Model file for the job. Use its own axes, mm. Give positions to 0.01 mm unless a question says otherwise; leave off trailing zeros. Loops run counter-clockwise (first coordinate to the right, second up) from the corner with the lowest first, then second, coordinate; pieces in that order, holes last. Notation, with made-up numbers: M -30,-19 L 10,-19 A11 cw 10,-14 Z; hole C 78,-34 d10. An arc over 180 degrees is marked long. Use CSV: the item, a comma, the result in double quotes. Start each with the question number.
(1) Flat gauge pin, fed straight in: P1, Ø1.7, axis at y = 46.375, z = -34.305, coming from the -X side. Where does the tip first touch, or does it go through?
(2) Slice it at B-B on y = 10.5. List the corners of the cut face in (x, z), and give its area (3 significant figures).
(3) Two-plate mould, pull along Z, no slides. Class faces 1 (the face through (0.986, 45.224, -33.423)), 2 (the face through (0.99, 21.24, -21.91)), 3 (the face through (0.99, -12.63, -13.88)): pulls with the +Z half, pulls with the -Z half, needs draft (parallel to the pull), parting line crosses it, or undercut.
(4) Slice it at C-C on z = -26. List the corners of the cut face in (x, y).
(5) Slice it at A-A on x = 1.05. List the corners of the cut face in (y, z) (3 decimals), and give its area (3 significant figures).
(6) Wall check: line 1 along Z through (x, y) = (0.35, -9.5); line 2 along Z through (x, y) = (0.95, 47.5); line 3 along Z through (x, y) = (0.7, 10.5). Give the ranges that are in metal, low to high. Write a range as from..to.
Solid Edge part; units mm, degrees
sketch "Sketch1" plane through (0, 0, 0) normal (1, 0, 0) x (0, 1, 0)
  arc A0 (-7.125, -12.3409) -> (-11.125, -19.2691) centre (-9.125, -15.805) ccw
  arc A1 (-6.8931, -21.1553) -> (-11.125, -19.2691) centre (0, 0) cw
  line L0 (45.1358, -38.1082) -> (-6.8931, -21.1553)
  arc A2 (47.6142, -30.5018) -> (45.1358, -38.1082) centre (46.375, -34.305) cw
  line L1 (-4.4147, -13.5489) -> (47.6142, -30.5018)
  arc A3 (-4.4147, -13.5489) -> (-7.125, -12.3409) centre (0, 0) cw
  circle A4 centre (-9.125, -15.805) radius 2.2
  circle A5 centre (46.375, -34.305) radius 1.45
extrude "Protrusion1" add sketch "Sketch1" along normal blind 2
Reply:
1,P1,"passes through"
2,outline,"M 0,-26.82 L 2,-26.82 L 2,-18.41 L 0,-18.41 Z"
2,area,"16.8 mm^2"
3,face 1,"undercut"
3,face 2,"pulls with the +Z half"
3,face 3,"parting line crosses it"
4,outline,"M 0,7.98 L 2,7.98 L 2,33.8 L 0,33.8 Z"
5,outline,"M -11.125,-19.269 A22.25 ccw -6.893,-21.155 L 45.136,-38.108 A4 ccw 47.614,-30.502 L -4.415,-13.549 A14.25 cw -7.125,-12.341 A4 ccw Z; hole C -9.125,-15.805 d4.4; hole C 46.375,-34.305 d2.9"
5,area,"497 mm^2"
6,line 1,"z = -20.12..-17.97, -13.64..-11.82"
6,line 2,"z = -38.14..-35.22, -33.39..-30.46"
6,line 3,"z = -26.82..-18.41"
